```python
from build123d import *

# Parameters (mm, degrees)
SZKIC1_R                    = 1.25
DODANIE_WYCI_GNI_CIE1_DEPTH = 8


with BuildPart() as part:
    # Szkic1 → Dodanie-wyciągnięcie1 (new body)
    with BuildSketch(Plane.XY):
        with BuildLine():
            Line((0.216930458, 0.048206768), (3.340774171, 0.74239426))
            ThreePointArc((3.340774171, 0.74239426), (4.010273516, 1.255718269), (4.04887337, 2.098476219))
            Line((4.04887337, 2.098476219), (1.633372376, 7.980129441))
            ThreePointArc((1.633372376, 7.980129441), (1.424945236, 8.297716323), (1.113109988, 8.514654282))
            ThreePointArc((1.113109988, 8.514654282), (0, 8.75), (-1.113109988, 8.514654282))
            ThreePointArc((-1.113109988, 8.514654282), (-1.424945236, 8.297716323), (-1.633372376, 7.980129441))
            Line((-1.633372376, 7.980129441), (-4.04887337, 2.098476219))
            ThreePointArc((-4.04887337, 2.098476219), (-4.010273516, 1.255718269), (-3.340774171, 0.74239426))
            Line((-3.340774171, 0.74239426), (-0.216930458, 0.048206768))
            ThreePointArc((-0.216930458, 0.048206768), (0, 0.024393829), (0.216930458, 0.048206768))
        make_face()
        with Locations((0, 6)):
            Circle(SZKIC1_R, mode=Mode.SUBTRACT)
    extrude(amount=DODANIE_WYCI_GNI_CIE1_DEPTH)


solid = part.part
```
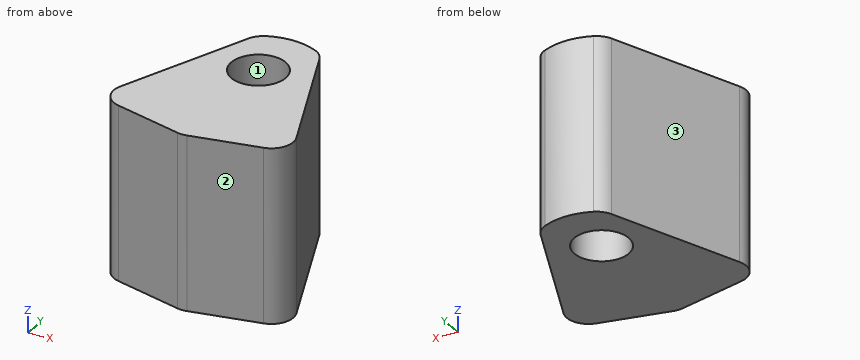
Verification items for the finished model (mm, model axes). Face numbers are marked on the shaded views. Coordinates: 2 decimals unless noted, no trailing zeros. Loops run counter-clockwise (first coordinate to the right, second up) from the corner with the lowest first, then second, coordinate; pieces in that order, holes last. Notation, with made-up numbers: (20.25, 18.5) -> (57.25, 18.5) arc R27 cw to (57.25, 34.5) -> close; hole circle Ø6 at (84, 31.25). An arc over 180 degrees is marked (long way). Answer in a Markdown table with one row per item.
1) Section check B-B (z = 6). Record the cut outline in (x, y).
The answers:
| item | result |
|---|---|
| outline | (-4.05, 2.1) arc R1 ccw to (-3.34, 0.74) -> (-0.22, 0.05) arc R1 ccw to (0.22, 0.05) -> (3.34, 0.74) arc R1 ccw to (4.05, 2.1) -> (1.63, 7.98) arc R1 ccw to (1.11, 8.51) arc R2.75 ccw to (-1.11, 8.51) arc R1 ccw to (-1.63, 7.98) -> close; hole circle Ø2.5 at (0, 6) |
2) Draft check along X on the marked faces 1, 2 and 3. Enter one of: released by +X, released by -X, zero draft, split by the parting line, or undercut.
The answers:
| item | result |
|---|---|
| face 1 | undercut |
| face 2 | released by +X |
| face 3 | released by -X |
3) Section check C-C (y = 6). Record the cut outline in (x, z).
The answers:
| item | result |
|---|---|
| outline | (-2.45, 0) -> (-1.25, 0) -> (-1.25, 8) -> (-2.45, 8) -> close; (1.25, 0) -> (2.45, 0) -> (2.45, 8) -> (1.25, 8) -> close |
4) Section check A-A (x = 0). Record the cut outline in (y, z), and give its area (3 significant figures).
The answers:
| item | result |
|---|---|
| outline | (0.02, 0) -> (4.75, 0) -> (4.75, 8) -> (0.02, 8) -> close; (7.25, 0) -> (8.75, 0) -> (8.75, 8) -> (7.25, 8) -> close |
| area | 49.8 mm2 |
5) Depth check by flat-ended pin: P1, Ø1, axis at y = 8, z = 2.5, coming from the -X side; P2, Ø2, axis at y = 7, z = 3, coming from the -X side; P3, Ø1, axis at y = 3, z = 2.5, coming from the +X side; P4, Ø1.5, axis at x = -0.5, y = 3.5, coming from the -Z side. Enter the tip coordinate at first touch or a pass-through.
The answers:
| item | result |
|---|---|
| P1 | stops at x = -1.83 |
| P2 | stops at x = -2.45 |
| P3 | stops at x = 3.88 |
| P4 | stops at z = 0 |
6) Section check D-D (x = -3). Record the cut outline in (y, z), and give its area (3 significant figures).
The answers:
| item | result |
|---|---|
| outline | (0.67, 0) -> (4.65, 0) -> (4.65, 8) -> (0.67, 8) -> close |
| area | 31.9 mm2 |
7) Scan lines: line 1 along X through (y, z) = (7, 3.25); line 2 along X through (y, z) = (6.5, 3.75); line 3 along X through (y, z) = (3.75, 4.75). Record each from-to range of solid material in increasing order. Write a range as from..to.
The answers:
| item | result |
|---|---|
| line 1 | x = -2.04..-0.75, 0.75..2.04 |
| line 2 | x = -2.24..-1.15, 1.15..2.24 |
| line 3 | x = -3.37..3.37 |
